```python
from build123d import *

# Parameters (mm, degrees)
F0_R     = 5
F1_DEPTH = 76.2
F2_R     = 12.5
F2_R_2   = 5
F3_DEPTH = 10.16
F4_R     = 8.89


with BuildPart() as f1:
    # F0 (on Top) → F1 (new body)
    with BuildSketch(Plane.XY):
        Circle(F0_R)
    extrude(amount=F1_DEPTH)

    # F2 (on face) → F3 (join)
    with BuildSketch(Plane.XY.offset(76.2)):
        Circle(F2_R)
        Circle(F2_R_2, mode=Mode.SUBTRACT)
        Circle(F2_R_2)
    extrude(amount=F3_DEPTH)

    # F4
    f4_edges = [f1.edges().sort_by_distance(p)[0] for p in [
        (-12.5, 0, 86.36),
    ]]
    fillet(f4_edges, radius=F4_R)


solid = f1.part
```
The model under review builds one solid part; all positions refer to its coordinate system, in mm. A direction names the side the tool comes from. Give positions to 0.01 mm unless a question says otherwise; leave off trailing zeros. Loops run counter-clockwise (first coordinate to the right, second up) from the corner with the lowest first, then second, coordinate; pieces in that order, holes last. Notation, with made-up numbers: (66.25, 25.25) - (98.25, 25.25) arc R11 cw to (98.25, 34.25) - close; hole circle Ø7 at (79.25, 37). An arc over 180 degrees is marked (long way). Answer as a JSON object with one key per item and string values.
Q1. Insertion check: pin 1 (4 mm diameter, centred on y = 1, z = 72.5, fed in from -X); pin 2 (4 mm diameter, centred on y = 1, z = 42, fed in from +X); pin 3 (8 mm diameter, centred on x = 3.5, z = 9, fed in from -Y). Each pin has a flat end and moves straight along its axis. Give the tip position at first contact, or say it passes through.
Worked out:
{"pin 1": "stops at x = -5", "pin 2": "stops at x = 5", "pin 3": "stops at y = -5"}
Q2. For faces 1 (the flat face through (0, 0, 0)), 2 (the flat face through (-0.2, -5.4, 76.2)), list the 3-axis set-ups (+Z, -Z, +X, -X, +Y, -Y) from which the entire face can be reached by the end or side of a thin tool; tool diameter is ignored.
Worked out:
{"face 1": "-Z, +X, -X, +Y, -Y", "face 2": "-Z"}
Q3. Add section A-A on z = 53. State the section outline as (x, y) points.
Worked out:
{"outline": "circle Ø10 at (0, 0)"}
Q4. To check wall thickness, follow line 1 along Y through (x, z) = (0.25, 41); line 2 along Z through (x, y) = (3.25, 1.75); line 3 along Y through (x, z) = (-1, 9). State the ranges of each line that lie inside material, in increasing order.
Worked out:
{"line 1": "y = -4.99 to 4.99", "line 2": "z = 0 to 86.36", "line 3": "y = -4.9 to 4.9"}
